from build123d import *

# Parameters (mm, degrees)
SKETCH2_W                   = 33.3375
SKETCH2_H                   = 12.7
F_12_0_189_DIAMETER_HOLE1_D = 4.8006
CIRPATTERN3_COUNT           = 6
CUT_EXTRUDE1_DEPTH          = 13.7
FILLET1_R                   = 4
CIRPATTERN4_COUNT           = 6
FILLET1_OF_CIRPATTERN4_R    = 4
CHAMFER1_SIZE               = 1
CHAMFER2_SIZE               = 1


with BuildPart() as part:
    # Sketch2 → Revolve1 (revolve)
    with BuildSketch(Plane(origin=(0, 0, 0), x_dir=(0, 0, -1), z_dir=(1, 0, 0))):
        with Locations((-65.88125, 6.35)):
            Rectangle(SKETCH2_W, SKETCH2_H)
    revolve(axis=Axis((0, -0.635, 0), (0, 1, 0)))

    # #12 (0.189) Diameter Hole1 (through all)
    with Locations(Plane(origin=(0, 12.7, 0), x_dir=(1, 0, 0), z_dir=(0, 1, 0))):
        with Locations((-35, 60.621778)):
            f_12_0_189_diameter_hole1 = Hole(F_12_0_189_DIAMETER_HOLE1_D / 2)

    # CirPattern3: #12 (0.189) Diameter Hole1 ×6 about axis
    cirpattern3_axis = Axis((0, 0, 0), (0, 1, 0))
    for i in range(1, CIRPATTERN3_COUNT):
        add(f_12_0_189_diameter_hole1.rotate(cirpattern3_axis, i * 360 / CIRPATTERN3_COUNT), mode=Mode.SUBTRACT)

    # Sketch8 → Cut-Extrude1 (cut, through all)
    with BuildSketch(Plane(origin=(0, 12.7, 0), x_dir=(1, 0, 0), z_dir=(0, 1, 0))):
        with BuildLine():
            Line((-22.66059, 49.249293), (-34.364196, 69.520533))
            ThreePointArc((-34.364196, 69.520533), (0, 77.55), (34.364196, 69.520533))
            Line((34.364196, 69.520533), (22.66059, 49.249293))
            ThreePointArc((22.66059, 49.249293), (0, 54.2125), (-22.66059, 49.249293))
        make_face()
    cut_extrude1 = extrude(amount=-CUT_EXTRUDE1_DEPTH, mode=Mode.SUBTRACT)

    # Fillet1
    fillet1_edges = [part.edges().sort_by_distance(p)[0] for p in [
        (22.66059, 6.35, -49.249293),
        (-22.66059, 6.35, -49.249293),
        (-34.364196, 6.35, -69.520533),
        (34.364196, 6.35, -69.520533),
    ]]
    fillet(fillet1_edges, radius=FILLET1_R)

    # CirPattern4: Cut-Extrude1 ×6 about axis
    cirpattern4_axis = Axis((0, 0, 0), (0, 1, 0))
    for i in range(1, CIRPATTERN4_COUNT):
        add(cut_extrude1.rotate(cirpattern4_axis, i * 360 / CIRPATTERN4_COUNT), mode=Mode.SUBTRACT)

    # Fillet1 of CirPattern4
    fillet1_of_cirpattern4_edges = [part.edges().sort_by_distance(p)[0] for p in [
        (-31.320844, 6.35, -44.249293),
        (-53.981433, 6.35, -5),
        (-77.388646, 6.35, -5),
        (-43.02445, 6.35, -64.520533),
        (-53.981433, 6.35, 5),
        (-31.320844, 6.35, 44.249293),
        (-43.02445, 6.35, 64.520533),
        (-77.388646, 6.35, 5),
        (-22.66059, 6.35, 49.249293),
        (22.66059, 6.35, 49.249293),
        (34.364196, 6.35, 69.520533),
        (-34.364196, 6.35, 69.520533),
        (31.320844, 6.35, 44.249293),
        (53.981433, 6.35, 5),
        (77.388646, 6.35, 5),
        (43.02445, 6.35, 64.520533),
        (53.981433, 6.35, -5),
        (31.320844, 6.35, -44.249293),
        (43.02445, 6.35, -64.520533),
        (77.388646, 6.35, -5),
    ]]
    fillet(fillet1_of_cirpattern4_edges, radius=FILLET1_OF_CIRPATTERN4_R)

    # Chamfer1
    chamfer1_edges = [part.edges().sort_by_distance(p)[0] for p in [
        (0, 12.7, -49.2125),
        (0, 0, -49.2125),
    ]]
    chamfer(chamfer1_edges, length=CHAMFER1_SIZE)

    # Chamfer2
    chamfer2_edges = [part.edges().sort_by_distance(p)[0] for p in [
        (0, 12.7, -82.55),
        (0, 0, -82.55),
    ]]
    chamfer(chamfer2_edges, length=CHAMFER2_SIZE)


solid = part.part
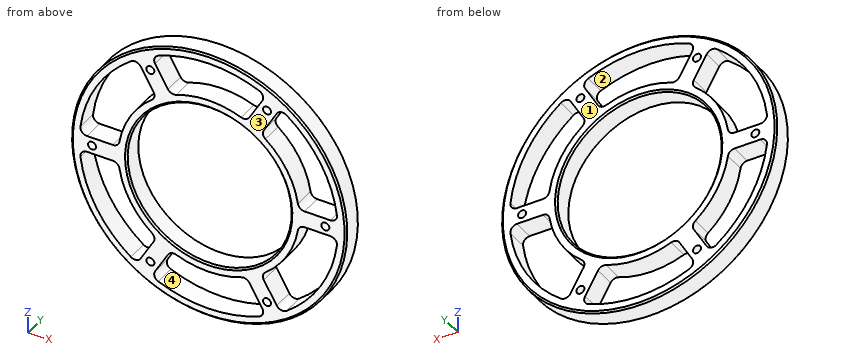
Check sheet for the modelled part. Datum: model origin and axes. Units: mm. Face numbers are marked on the shaded views. A direction names the side the tool comes from. Coordinates: 2 decimals unless noted, no trailing zeros. Loops run counter-clockwise (first coordinate to the right, second up) from the corner with the lowest first, then second, coordinate; pieces in that order, holes last. Notation, with made-up numbers: (-22.5, 66) -> (28.5, 66) arc R17 cw to (28.5, 85) -> close; hole circle Ø1 at (9.25, 55). An arc over 180 degrees is marked (long way). Answer in a Markdown table with one row per item.
1. Sectioned sample at A-A, the plane x = 0. Record the boundary of the cut face in (y, z), then the cut area to 3 significant figures.
Check values:
| item | result |
|---|---|
| outline | (0, -81.55) -> (1, -82.55) -> (11.7, -82.55) -> (12.7, -81.55) -> (12.7, -77.55) -> (0, -77.55) -> close; (0, -54.21) -> (12.7, -54.21) -> (12.7, -50.21) -> (11.7, -49.21) -> (1, -49.21) -> (0, -50.21) -> close; (0, 50.21) -> (1, 49.21) -> (11.7, 49.21) -> (12.7, 50.21) -> (12.7, 54.21) -> (0, 54.21) -> close; (0, 77.55) -> (12.7, 77.55) -> (12.7, 81.55) -> (11.7, 82.55) -> (1, 82.55) -> (0, 81.55) -> close |
| area | 250 mm2 |
2. Sectioned sample at C-C, the plane y = 4.5. Give the number of separate pieces and of enclosed holes in the cut face, then the cut area to 3 significant figures.
Check values:
| item | result |
|---|---|
| separate pieces | 1 |
| enclosed holes | 13 |
| area | 5,510 mm2 |
3. Go/stop test with flat-tipped pins: pin 1 (5 mm diameter, centred on x = 41.5, y = 5.5, fed in from -Z); pin 2 (4 mm diameter, centred on x = 35, z = 60.62, fed in from -Y); pin 3 (2 mm diameter, centred on y = 11, z = 39.5, fed in from +X); pin 4 (2 mm diameter, centred on x = -43, y = 11, fed in from +Z). Record where each tip stops, or that it passes through.
Check values:
| item | result |
|---|---|
| pin 1 | stops at z = -72.76 |
| pin 2 | passes through |
| pin 3 | stops at x = 73.02 |
| pin 4 | stops at z = 71.07 |
4. Sectioned sample at B-B, the plane z = 0. Record the boundary of the cut face in (x, y), then the cut area to 3 significant figures.
Check values:
| item | result |
|---|---|
| outline | (-82.55, 1) -> (-81.55, 0) -> (-72.4, 0) -> (-72.4, 12.7) -> (-81.55, 12.7) -> (-82.55, 11.7) -> close; (-67.6, 0) -> (-50.21, 0) -> (-49.21, 1) -> (-49.21, 11.7) -> (-50.21, 12.7) -> (-67.6, 12.7) -> close; (49.21, 1) -> (50.21, 0) -> (67.6, 0) -> (67.6, 12.7) -> (50.21, 12.7) -> (49.21, 11.7) -> close; (72.4, 0) -> (81.55, 0) -> (82.55, 1) -> (82.55, 11.7) -> (81.55, 12.7) -> (72.4, 12.7) -> close |
| area | 721 mm2 |
5. Release check for a two-part mould opening along X. For the marked faces 1 and 2 record: released by +X, released by -X, zero draft, split by the parting line, or undercut.
Check values:
| item | result |
|---|---|
| face 1 | zero draft |
| face 2 | undercut |
6. Access from +Z, -Z, +X, -X, +Y, -Y to the whole of each face (thin tool, end or side, straight path). Record for the marked faces 3 and 4.
Check values:
| item | result |
|---|---|
| face 3 | +Z, -Z, +X, -X, -Y |
| face 4 | +Y, -Y |
7. Material ranges on line 1 along X through (y, z) = (10.5, -55.5); line 2 along X through (y, z) = (12, -56); line 3 along Z through (x, y) = (-35, 2.5), recorded low to high. Write a range as [from, to].
Check values:
| item | result |
|---|---|
| line 1 | x = [-61.11, -54.16], [-37.82, -26.27], [26.27, 37.82], [54.16, 61.11] |
| line 2 | x = [-60.24, -53.65], [-38.11, -26.56], [26.56, 38.11], [53.65, 60.24] |
| line 3 | z = [-74.76, -63.02], [-58.22, -50.62], [-41.4, -34.6], [34.6, 41.4], [50.62, 58.22], [63.02, 74.76] |
